Geometry check sheet. Reference: the model listing, model coordinates, mm. A direction names the side the tool comes from. Round coordinates to 2 decimals unless told otherwise and drop trailing zeros. Write each loop counter-clockwise with the first axis right and the second up, starting at its lowest first coordinate (ties: lowest second). Pieces come first, ordered by that corner, then holes.
from build123d import *

# Parameters (mm, degrees)
F0_R     = 11
F1_DEPTH = 14
F3_DEPTH = 7
F5_DEPTH = 7
F7_DEPTH = 7


with BuildPart() as f1:
    # F0 (on Top) → F1 (new body)
    with BuildSketch(Plane.XY):
        with BuildLine():
            ThreePointArc((21.5405989438, -14.4337567297), (19.7489488314, -6.9989706734), (16.6666666667, 0))
            Line((16.6666666667, 0), (12.5, 7.2168783649))
            Line((12.5, 7.2168783649), (1.7297019, 25.8715818867))
            ThreePointArc((1.7297019, 25.8715818867), (-3.8131871995, 20.6025755779), (-8.3333333333, 14.4337567297))
            Line((-8.3333333333, 14.4337567297), (-12.5, 7.2168783649))
            Line((-12.5, 7.2168783649), (-23.2702981, -11.437825157))
            ThreePointArc((-23.2702981, -11.437825157), (-15.9357602341, -13.6036047731), (-8.3333333333, -14.4337567297))
            Line((-8.3333333333, -14.4337567297), (0, -14.4337567297))
            Line((0, -14.4337567297), (21.5405989438, -14.4337567297))
        make_face()
        Circle(F0_R, mode=Mode.SUBTRACT)
    extrude(amount=F1_DEPTH)

    # F2 (on face) → F3 (cut)
    with BuildSketch(Plane(origin=(12.5, 7.2168783649, 0), x_dir=(-0.5, 0.8660254038, 0), z_dir=(0.8660254038, 0.5, 0))):
        Polygon((19.5405962, 4.1867693368), (19.5405962, 9.9602720287), (14.5405962, 12.8470233746), (9.5405962, 9.9602720287), (9.5405962, 4.1867693368), (14.5405962, 1.3000179909), align=None)
    extrude(amount=-F3_DEPTH, mode=Mode.SUBTRACT)

    # F4 (on face) → F5 (cut)
    with BuildSketch(Plane.XZ.offset(14.4337567297)):
        Polygon((19.5405989438, 4.1132486541), (19.5405989438, 9.8867513459), (14.5405989438, 12.7735026919), (9.5405989438, 9.8867513459), (9.5405989438, 4.1132486541), (14.5405989438, 1.2264973081), align=None)
    extrude(amount=-F5_DEPTH, mode=Mode.SUBTRACT)

    # F6 (on face) → F7 (cut)
    with BuildSketch(Plane(origin=(-12.5, 7.2168783649, 0), x_dir=(-0.5, -0.8660254038, 0), z_dir=(-0.8660254038, 0.5, 0))):
        Polygon((19.5405962, 4.1132486541), (19.5405962, 9.8867513459), (14.5405962, 12.7735026919), (9.5405962, 9.8867513459), (9.5405962, 4.1132486541), (14.5405962, 1.2264973081), align=None)
    extrude(amount=-F7_DEPTH, mode=Mode.SUBTRACT)


solid = f1.part
1. Section check A-A (z = 8.5). Record the cut outline in (x, y).
2. Scan lines: line 1 along Y through (x, z) = (0, 9.5); line 2 along Y through (x, z) = (-1, 3); line 3 along Z through (x, y) = (1, 18.5). Record each from-to range of solid material in increasing order.
3. Release check for a two-part mould opening along X. For faces 1 (the face through (-16.041, -13.582, 6.902)), 2 (the face through (-15.549, -4.966, 11.35)), 3 (the face through (-0.8, 16.25, 7.15)), 4 (the face through (3, -14.434, 7)) record: +X half, -X half, draft (parallel to the pull), parting line (faces both ways), or undercut.
4. Depth check by flat-ended pin: pin 1 Ø3 at (y, z) = (2, 10.5) entering from -X; pin 2 Ø3 at (y, z) = (4.5, 11) entering from -X; pin 3 Ø4 at (y, z) = (-4.5, 8.5) entering from +X; pin 4 Ø17.5 at (x, y) = (0, 0) entering from +Z. Enter the tip coordinate at first touch or a pass-through.
5. Section check B-B (x = 9). Record the cut outline in (y, z), plus the area to 3 significant figures.
6. Section check D-D (y = -4). Record the cut outline in (x, z).
7. Access from +Z, -Z, +X, -X, +Y, -Y to the whole of each face (thin tool, end or side, straight path). Record for faces 5 (the face through (-2.38, -10.74, 6.9)), 6 (the face through (-0.259, 22.414, 7.033)), 7 (the face through (0.97, 20.28, 11.38)), 8 (the face through (-3.742, 20.683, 6.902)), 9 (the face through (-14.28, -2.77, 7.04)).
8. Section check C-C (x = 0). Record the cut outline in (y, z).
Results below:
1. outline: (-23.27, -11.44) arc R42.93 ccw to (-8.33, -14.43) - (9.54, -14.43) - (9.54, -7.43) - (19.54, -7.43) - (19.54, -14.43) - (21.54, -14.43) arc R42.93 ccw to (16.67, 0) - (7.73, 15.48) - (1.67, 11.98) - (-3.33, 20.64) - (2.73, 24.14) - (1.73, 25.87) arc R42.93 ccw to (-8.33, 14.43) - (-17.27, -1.05) - (-11.21, -4.55) - (-16.21, -13.21) - (-22.27, -9.71) - close; hole circle Ø22 at (0, 0)
2. line 1: y = -14.43 to -11, 11 to 14.87, 22.56 to 24.42
2. line 2: y = -14.43 to -10.95, 10.95 to 16.6, 19.61 to 23.51
2. line 3: z = 0 to 1.87, 12.28 to 14
3. face 1: -X half
3. face 2: undercut
3. face 3: undercut
3. face 4: draft
4. pin 1: stops at x = -16.38
4. pin 2: stops at x = -14.93
4. pin 3: stops at x = 19.58
4. pin 4: passes through
5. outline: (-14.43, 0) - (-6.32, 0) - (-6.32, 14) - (-14.43, 14) - close; (6.32, 0) - (13.28, 0) - (13.28, 14) - (6.32, 14) - close
5. area: 211 mm2
6. outline: (-18.98, 0) - (-10.25, 0) - (-10.25, 14) - (-18.98, 14) - (-18.98, 11.86) - (-12.15, 9.89) - (-12.15, 4.11) - (-18.98, 2.14) - close; (10.25, 0) - (18.61, 0) - (18.61, 14) - (10.25, 14) - close
7. face 5: +Z, -Z
7. face 6: +X
7. face 7: none
7. face 8: +Z, -Z, -X, +Y
7. face 9: -X
8. outline: (-14.43, 0) - (-11, 0) - (-11, 14) - (-14.43, 14) - close; (11, 0) - (24.42, 0) - (24.42, 14) - (11, 14) - close; hole (14.87, 2.26) - (16.79, 1.3) - (22.56, 4.19) - (22.56, 9.96) - (16.79, 12.85) - (14.87, 11.89) - close
